```python
from build123d import *

# Parameters (mm, degrees)
F3_DEPTH = 7
F5_DEPTH = 7


with BuildPart() as f1:
    # F0 (on Front) → F1 (revolve)
    with BuildSketch(Plane.XZ):
        with BuildLine():
            Line((0, 13.4), (0, 0))
            Line((0, 0), (44.5, 0))
            Line((44.5, 0), (44.5, 9.9))
            add(Edge.make_bspline(
                [(0, 13.4), (2.9930189026, 13.4), (23.6956200801, 13.1516238506), (36.554730518, 11.2935173538), (44.5, 9.9)],
                knots=[0, 0, 0, 0, 0.48923543, 1, 1, 1, 1], degree=3))
        make_face()
        with BuildLine():
            Line((-44.5, 0), (0, 0))
            Line((0, 0), (0, 13.4))
            add(Edge.make_bspline(
                [(0, 13.4), (-2.9930189026, 13.4), (-23.6956200801, 13.1516238506), (-36.554730518, 11.2935173538), (-44.5, 9.9)],
                knots=[0, 0, 0, 0, 0.48923543, 1, 1, 1, 1], degree=3))
            Line((-44.5, 9.9), (-44.5, 0))
        make_face()
    revolve(axis=Axis((22.25, 0, 0), (1, 0, 0)))

    # F2 (on face) → F3 (cut)
    with BuildSketch(Plane(origin=(-44.5, 0, 0), x_dir=(0, -1, 0), z_dir=(-1, 0, 0))):
        Polygon((-3.8249455334, -6.625), (3.8249455334, -6.625), (7.6498910668, 0), (3.8249455334, 6.625), (-3.8249455334, 6.625), (-7.6498910668, 0), align=None)
    extrude(amount=-F3_DEPTH, mode=Mode.SUBTRACT)

    # F4 (on face) → F5 (cut)
    with BuildSketch(Plane.YZ.offset(44.5)):
        Polygon((-3.8249455334, -6.625), (3.8249455334, -6.625), (7.6498910668, 0), (3.8249455334, 6.625), (-3.8249455334, 6.625), (-7.6498910668, 0), align=None)
    extrude(amount=-F5_DEPTH, mode=Mode.SUBTRACT)


solid = f1.part
```
Model file for the job. Use its own axes, mm. A direction names the side the tool comes from. Give positions to 0.01 mm unless a question says otherwise; leave off trailing zeros. Use a Markdown table: item, result.
1) Pin check, flat tips, straight feed: pin 1 (1.5 mm diameter, centred on x = -10.5, z = 7, fed in from -Y); pin 2 (6.5 mm diameter, centred on y = -2, z = 2.5, fed in from +X); pin 3 (3.5 mm diameter, centred on x = 42, y = -1.5, fed in from -Z). Stop position of each tip, or through.
Responses:
| item | result |
|---|---|
| pin 1 | stops at y = -11.66 |
| pin 2 | stops at x = 37.5 |
| pin 3 | stops at z = -10.57 |
2) Tool access for faces 1 (the flat face through (-37.5, 0, 0)), 2 (the flat face through (41.05, 5.71, -3.36)), 3 (the flat face through (-44.5, 6.5, -2.3)): list every direction of +Z, -Z, +X, -X, +Y, -Y with a clear straight run to the whole face (end or side of a thin tool).
Responses:
| item | result |
|---|---|
| face 1 | -X |
| face 2 | +X |
| face 3 | +Z, -Z, -X, +Y, -Y |
3) Drill centre lines: line 1 (X direction, y = -5, z = 1.25); line 2 (Y direction, x = -40, z = 3.25); line 3 (Z direction, x = 17, y = 7.5). Where is each one in solid material? Low to high. Write a range as from..to.
Responses:
| item | result |
|---|---|
| line 1 | x = -37.5..37.5 |
| line 2 | y = -10.15..-5.77, 5.77..10.15 |
| line 3 | z = -10.62..10.62 |
4) Pull direction Z, two halves, no side cores. Call faces 4 (the flat face through (44.5, 6.5, 2.3)), 5 (the flat face through (-41.05, -5.71, -3.36)): +Z half, -Z half, draft (parallel to the pull), parting line (faces both ways), or undercut.
Responses:
| item | result |
|---|---|
| face 4 | draft |
| face 5 | undercut |
